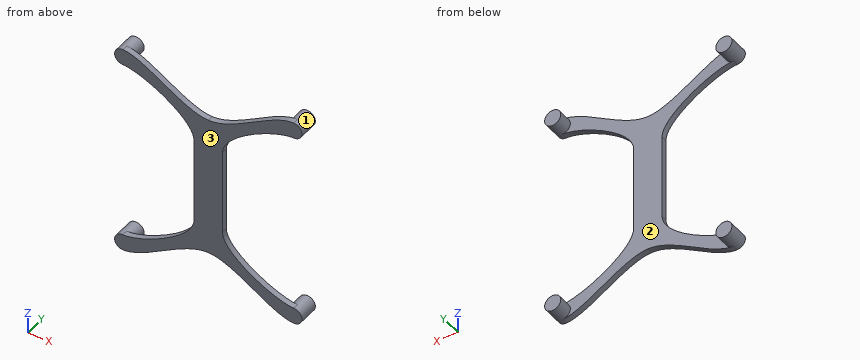
from build123d import *

# Parameters (mm, degrees)
BOSS_EXTRUDE1_DEPTH                        = 2.54
SKETCH2_R                                  = 3.594100000000004
BOSS_EXTRUDE2_DEPTH                        = 6.35
MIRROR1_AT_THE_SECOND_PLANE_COPY_1_DEPTH   = 2.54
MIRROR1_AT_THE_SECOND_PLANE_COPY_2_SKETC_R = 3.594100000000004
MIRROR1_AT_THE_SECOND_PLANE_COPY_2_DEPTH   = 6.35


with BuildPart() as part:
    # Sketch1 → Boss-Extrude1 (new body)
    with BuildSketch(Plane(origin=(0, 0, 0), x_dir=(1, 0, 0), z_dir=(0, 1, 0))):
        with BuildLine():
            Line((-6.35, -7.8e-16), (0, 0))
            Line((0, 0), (0, 31.75))
            add(Edge.make_bspline(
                [(0, 31.75), (-11.909179237119448, 31.827130893047123), (-27.615811236602134, 47.867470834719654), (-38.01020913703169, 48.0429782090805)],
                knots=[0, 0, 0, 0, 0.9971245716363047, 0.9971245716363047, 0.9971245716363047, 0.9971245716363047], degree=3))
            ThreePointArc((-38.01020913703169, 48.0429782090805), (-35.52703749049909, 46.95946582656603), (-34.5059, 44.44999999999999))
            ThreePointArc((-34.5059, 44.44999999999999), (-35.55858751773743, 41.908587517737416), (-38.1, 40.855899999999984))
            add(Edge.make_bspline(
                [(-6.35, 19.05), (-6.175250797111612, 28.394037165914764), (-28.752700179166496, 40.793112384563265), (-38.1, 40.855899999999984)],
                knots=[0, 0, 0, 0, 1, 1, 1, 1], degree=3))
            Line((-6.35, 19.05), (-6.35, -7.8e-16))
        make_face()
        with BuildLine():
            add(Edge.make_bspline(
                [(-38.01020913703169, 48.0429782090805), (-38.04018367320963, 48.043484323257836), (-38.07011403368422, 48.04385850798247), (-38.100000000000016, 48.04409999999999)],
                knots=[0.9971245716363047, 0.9971245716363047, 0.9971245716363047, 0.9971245716363047, 1, 1, 1, 1], degree=3))
            ThreePointArc((-38.01020913703169, 48.0429782090805), (-38.05510106491391, 48.04381954132759), (-38.100000000000016, 48.04409999999999))
        make_face()
        with BuildLine():
            ThreePointArc((-34.5059, 44.44999999999999), (-35.52703749049909, 46.95946582656603), (-38.01020913703169, 48.0429782090805))
            add(Edge.make_bspline(
                [(-38.01020913703169, 48.0429782090805), (-38.04018367320963, 48.043484323257836), (-38.07011403368422, 48.04385850798247), (-38.100000000000016, 48.04409999999999)],
                knots=[0.9971245716363047, 0.9971245716363047, 0.9971245716363047, 0.9971245716363047, 1, 1, 1, 1], degree=3))
            ThreePointArc((-38.100000000000016, 48.04409999999999), (-41.694100000000006, 44.44999999999998), (-38.1, 40.855899999999984))
            ThreePointArc((-38.1, 40.855899999999984), (-35.55858751773743, 41.908587517737416), (-34.5059, 44.44999999999999))
        make_face()
    boss_extrude1 = extrude(amount=BOSS_EXTRUDE1_DEPTH)

    # Sketch2 → Boss-Extrude2 (add)
    with BuildSketch(Plane(origin=(0, 2.54, 0), x_dir=(1, 0, 0), z_dir=(0, 1, 0))):
        with Locations(Location((-38.1, 44.44999999999999, 0), (0, 0, 270))):
            Circle(SKETCH2_R)
    boss_extrude2 = extrude(amount=BOSS_EXTRUDE2_DEPTH)

    # Mirror1: Boss-Extrude1, Boss-Extrude2 across plane
    add(boss_extrude1.mirror(Plane(origin=(0, 0, 0), x_dir=(0, 0, 1), z_dir=(1, 0, 0))))
    add(boss_extrude2.mirror(Plane(origin=(0, 0, 0), x_dir=(0, 0, 1), z_dir=(1, 0, 0))))

    # Mirror1 at the second plane: Boss-Extrude1, Boss-Extrude2 across plane
    add(boss_extrude1.mirror(Plane.XY))
    add(boss_extrude2.mirror(Plane.XY))

    # Mirror1 at the second plane copy 1 sketc → Mirror1 at the second plane copy 1 (add)
    with BuildSketch(Plane(origin=(0, 0, 0), x_dir=(-1, 0, 0), z_dir=(0, 1, 0))):
        with BuildLine():
            Line((-6.35, -7.8e-16), (0, 0))
            Line((0, 0), (0, 31.75))
            add(Edge.make_bspline(
                [(0, 31.75), (-11.909179237119448, 31.827130893047123), (-27.615811236602134, 47.867470834719654), (-38.01020913703169, 48.0429782090805)],
                knots=[0, 0, 0, 0, 0.9971245716363047, 0.9971245716363047, 0.9971245716363047, 0.9971245716363047], degree=3))
            ThreePointArc((-38.01020913703169, 48.0429782090805), (-35.52703749049909, 46.95946582656603), (-34.5059, 44.44999999999999))
            ThreePointArc((-34.5059, 44.44999999999999), (-35.55858751773743, 41.908587517737416), (-38.1, 40.855899999999984))
            add(Edge.make_bspline(
                [(-6.35, 19.05), (-6.175250797111612, 28.394037165914764), (-28.752700179166496, 40.793112384563265), (-38.1, 40.855899999999984)],
                knots=[0, 0, 0, 0, 1, 1, 1, 1], degree=3))
            Line((-6.35, 19.05), (-6.35, -7.8e-16))
        make_face()
        with BuildLine():
            add(Edge.make_bspline(
                [(-38.01020913703169, 48.0429782090805), (-38.04018367320963, 48.043484323257836), (-38.07011403368422, 48.04385850798247), (-38.100000000000016, 48.04409999999999)],
                knots=[0.9971245716363047, 0.9971245716363047, 0.9971245716363047, 0.9971245716363047, 1, 1, 1, 1], degree=3))
            ThreePointArc((-38.01020913703169, 48.0429782090805), (-38.05510106491391, 48.04381954132759), (-38.100000000000016, 48.04409999999999))
        make_face()
        with BuildLine():
            ThreePointArc((-34.5059, 44.44999999999999), (-35.52703749049909, 46.95946582656603), (-38.01020913703169, 48.0429782090805))
            add(Edge.make_bspline(
                [(-38.01020913703169, 48.0429782090805), (-38.04018367320963, 48.043484323257836), (-38.07011403368422, 48.04385850798247), (-38.100000000000016, 48.04409999999999)],
                knots=[0.9971245716363047, 0.9971245716363047, 0.9971245716363047, 0.9971245716363047, 1, 1, 1, 1], degree=3))
            ThreePointArc((-38.100000000000016, 48.04409999999999), (-41.694100000000006, 44.44999999999998), (-38.1, 40.855899999999984))
            ThreePointArc((-38.1, 40.855899999999984), (-35.55858751773743, 41.908587517737416), (-34.5059, 44.44999999999999))
        make_face()
    extrude(amount=MIRROR1_AT_THE_SECOND_PLANE_COPY_1_DEPTH)

    # Mirror1 at the second plane copy 2 sketc → Mirror1 at the second plane copy 2 (add)
    with BuildSketch(Plane(origin=(0, 2.54, 0), x_dir=(-1, 0, 0), z_dir=(0, 1, 0))):
        with Locations(Location((-38.1, 44.44999999999999, 0), (0, 0, 270))):
            Circle(MIRROR1_AT_THE_SECOND_PLANE_COPY_2_SKETC_R)
    extrude(amount=MIRROR1_AT_THE_SECOND_PLANE_COPY_2_DEPTH)


solid = part.part
Design review of the part built by this model. Coordinates are the model's own, in mm. Face numbers are marked on the shaded views. Give positions to 0.01 mm unless a question says otherwise; leave off trailing zeros. Write each loop counter-clockwise with the first axis right and the second up, starting at its lowest first coordinate (ties: lowest second). Pieces come first, ordered by that corner, then holes. Notation, with made-up numbers: M -31,44.25 L -3,44.25 A18 ccw -3,63.25 Z; hole C -16.75,3 d3. An arc over 180 degrees is marked long. Answer as a JSON object with one key per item and string values. Group by question number.
1) Mouldability with a two-part tool opening along X and no side actions: class the marked faces 1, 2 and 3 as released by +X, released by -X, zero draft, split by the parting line, or undercut.
2) For line 1 along Z through (x, y) = (-0.5, 2.5); line 2 along Z through (x, y) = (-35, 4.5); line 3 along Z through (x, y) = (32, 1), list the stretches that pass through material, from the lowest coordinate up.
3) Clearance check with flat-ended pins moving along their axes: pin 1 Ø3 at (y, z) = (3.5, -32.5) entering from +X; pin 2 Ø2 at (y, z) = (0.5, 6.5) entering from -X; pin 3 Ø5 at (x, z) = (6, 35.5) entering from +Y. State where each tip first meets the part, or that it passes through.
4) We need section B-B (z = -17.5). Give the boundary of the cut face in (x, y), and give its area (3 significant figures).
5) We need section A-A (y = 5.75). Give the boundary of the cut face in (x, z).
Answer key:
{
 "1": {"face 1": "undercut", "face 2": "undercut", "face 3": "zero draft"},
 "2": {"line 1": "z = -31.76 to 31.76", "line 2": "z = -46.27 to -42.63, 42.63 to 46.27", "line 3": "z = -46.62 to -39.72, 39.72 to 46.62"},
 "3": {"pin 1": "stops at x = 19", "pin 2": "stops at x = -6.35", "pin 3": "stops at y = 2.54"},
 "4": {"outline": "M -6.35,0 L 6.35,0 L 6.35,2.54 L -6.35,2.54 Z", "area": "32.3 mm²"},
 "5": {"outline": "C -38.1,-44.45 d7.19; C -38.1,44.45 d7.19; C 38.1,-44.45 d7.19; C 38.1,44.45 d7.19"}
}
